Check sheet for the modelled part. Datum: model origin and axes. Units: mm. A direction names the side the tool comes from. Give positions to 0.01 mm unless a question says otherwise; leave off trailing zeros. Loops run counter-clockwise (first coordinate to the right, second up) from the corner with the lowest first, then second, coordinate; pieces in that order, holes last. Notation, with made-up numbers: (76, -24) - (87, -24) arc R19 cw to (87, 0) - close; hole circle Ø8 at (43.25, -23.75). An arc over 180 degrees is marked (long way). Use one line per item in the form item = value.
from build123d import *

# Parameters (mm, degrees)
SKETCH1_W           = 90
SKETCH1_H           = 80
BOSS_EXTRUDE1_DEPTH = 14
BOSS_EXTRUDE2_DEPTH = 1
SKETCH3_R           = 3.25
CUT_EXTRUDE1_DEPTH  = 111.613393245
SKETCH4_R           = 5.5
CUT_EXTRUDE2_DEPTH  = 7
SKETCH5_W           = 2
SKETCH5_H           = 6
SKETCH5_W_2         = 5
SKETCH5_H_2         = 5
CUT_EXTRUDE3_DEPTH  = 75
FILLET2_R           = 0.5
SKETCH6_R           = 1.5
CUT_EXTRUDE4_DEPTH  = 7
SKETCH7_R           = 1.5
CUT_EXTRUDE5_DEPTH  = 7
SKETCH8_W           = 12
SKETCH8_H           = 5
CUT_EXTRUDE6_DEPTH  = 5
SKETCH9_R           = 1.75
CUT_EXTRUDE7_DEPTH  = 111.09233745
SKETCH10_R          = 3
SKETCH10_R_2        = 3.25
CUT_EXTRUDE8_DEPTH  = 4
MOVE_FACE1_BY       = 0.2
MOVE_FACE1_2_BY     = 0.2
SKETCH11_W          = 10
SKETCH11_H          = 10
CUT_EXTRUDE10_DEPTH = 111.613393245


with BuildPart() as part:
    # Sketch1 → Boss-Extrude1 (new body)
    with BuildSketch(Plane(origin=(0, 0, 0), x_dir=(1, 0, 0), z_dir=(0, 1, 0))):
        with Locations((32.137715261, -38.032657583)):
            Rectangle(SKETCH1_W, SKETCH1_H)
    extrude(amount=BOSS_EXTRUDE1_DEPTH)

    # Sketch2 → Boss-Extrude2 (add)
    with BuildSketch(Plane(origin=(0, 14, 0), x_dir=(1, 0, 0), z_dir=(0, 1, 0))):
        Polygon((-12.862284739, -78.032657583), (77.137715261, -78.032657583), (77.137715261, -68.032657583), (77.137715261, 1.967342417), (70.137715261, 1.967342417), (70.137715261, -73.032657583), (-5.862284739, -73.032657583), (-5.862284739, 1.967342417), (-12.862284739, 1.967342417), (-12.862284739, -73.032657583), align=None)
    extrude(amount=BOSS_EXTRUDE2_DEPTH)

    # Sketch3 → Cut-Extrude1 (cut, through all)
    with BuildSketch(Plane(origin=(0, 14, 0), x_dir=(1, 0, 0), z_dir=(0, 1, 0))):
        with Locations(Location((57.137715261, -38.032657583, 0), (0, 0, 270))):
            Circle(SKETCH3_R)
        with Locations(Location((7.137715261, -38.032657583, 0), (0, 0, 270))):
            Circle(SKETCH3_R)
        with Locations(Location((7.137715261, -13.032657583, 0), (0, 0, 270))):
            Circle(SKETCH3_R)
        with Locations(Location((57.137715261, -13.032657583, 0), (0, 0, 270))):
            Circle(SKETCH3_R)
    extrude(amount=-CUT_EXTRUDE1_DEPTH, mode=Mode.SUBTRACT)

    # Sketch4 → Cut-Extrude2 (cut)
    with BuildSketch(Plane(origin=(0, 14, 0), x_dir=(1, 0, 0), z_dir=(0, 1, 0))):
        with Locations(Location((7.137715261, -38.032657583, 0), (0, 0, 270))):
            Circle(SKETCH4_R)
        with Locations(Location((57.137715261, -38.032657583, 0), (0, 0, 270))):
            Circle(SKETCH4_R)
        with Locations(Location((57.137715261, -13.032657583, 0), (0, 0, 270))):
            Circle(SKETCH4_R)
        with Locations(Location((7.137715261, -13.032657583, 0), (0, 0, 270))):
            Circle(SKETCH4_R)
    extrude(amount=-CUT_EXTRUDE2_DEPTH, mode=Mode.SUBTRACT)

    # Sketch5 → Cut-Extrude3 (cut)
    with BuildSketch(Plane(origin=(0, 0, -1.967342417), x_dir=(-1, 0, 0), z_dir=(0, 0, -1))):
        Polygon((-45.637715261, 14), (-43.637715261, 14), (-39.637715261, 10), (-49.637715261, 10), align=None)
        Polygon((-14.637715261, 10), (-24.637715261, 10), (-20.637715261, 14), (-18.637715261, 14), align=None)
        with Locations((-69.137715261, 11)):
            Rectangle(SKETCH5_W, SKETCH5_H)
        with Locations((4.862284739, 11)):
            Rectangle(SKETCH5_W, SKETCH5_H)
        with Locations((-32.137715261, 11.5)):
            Rectangle(SKETCH5_W_2, SKETCH5_H_2)
    extrude(amount=-CUT_EXTRUDE3_DEPTH, mode=Mode.SUBTRACT)

    # Fillet2
    fillet2_edges = [part.edges().sort_by_distance(p)[0] for p in [
        (68.137715261, 14, 35.532657583),
        (-3.862284739, 14, 35.532657583),
        (20.637715261, 14, 35.532657583),
        (18.637715261, 14, 35.532657583),
        (43.637715261, 14, 35.532657583),
        (45.637715261, 14, 35.532657583),
    ]]
    fillet(fillet2_edges, radius=FILLET2_R)

    # Sketch6 → Cut-Extrude4 (cut)
    with BuildSketch(Plane(origin=(77.137715261, 0, 0), x_dir=(0, 0, -1), z_dir=(1, 0, 0))):
        with Locations((-3.032657583, 12.5)):
            Circle(SKETCH6_R)
        with Locations((-13.032657583, 12.5)):
            Circle(SKETCH6_R)
        with Locations((-23.032657583, 12.5)):
            Circle(SKETCH6_R)
        with Locations((-33.032657583, 12.5)):
            Circle(SKETCH6_R)
        with Locations((-43.032657583, 12.5)):
            Circle(SKETCH6_R)
        with Locations((-53.032657583, 12.5)):
            Circle(SKETCH6_R)
        with Locations((-63.032657583, 12.5)):
            Circle(SKETCH6_R)
    extrude(amount=-CUT_EXTRUDE4_DEPTH, mode=Mode.SUBTRACT)

    # Sketch7 → Cut-Extrude5 (cut)
    with BuildSketch(Plane.ZY.offset(12.862284739)):
        with Locations((3.032657583, 11)):
            Circle(SKETCH7_R)
        with Locations((13.032657583, 11)):
            Circle(SKETCH7_R)
        with Locations((23.032657583, 11)):
            Circle(SKETCH7_R)
        with Locations((33.032657583, 11)):
            Circle(SKETCH7_R)
        with Locations((43.032657583, 11)):
            Circle(SKETCH7_R)
        with Locations((53.032657583, 11)):
            Circle(SKETCH7_R)
        with Locations((63.032657583, 11)):
            Circle(SKETCH7_R)
    extrude(amount=-CUT_EXTRUDE5_DEPTH, mode=Mode.SUBTRACT)

    # Sketch8 → Cut-Extrude6 (cut)
    with BuildSketch(Plane(origin=(0, 0, -1.967342417), x_dir=(-1, 0, 0), z_dir=(0, 0, -1))):
        with Locations((-32.137715261, 11.5)):
            Rectangle(SKETCH8_W, SKETCH8_H)
    extrude(amount=-CUT_EXTRUDE6_DEPTH, mode=Mode.SUBTRACT)

    # Sketch9 → Cut-Extrude7 (cut, through all)
    with BuildSketch(Plane(origin=(0, 9, 0), x_dir=(1, 0, 0), z_dir=(0, 1, 0))):
        with Locations(Location((36.137715261, -0.532657583, 0), (0, 0, 270))):
            Circle(SKETCH9_R)
        with Locations(Location((28.137715261, -0.532657583, 0), (0, 0, 90))):
            Circle(SKETCH9_R)
    extrude(amount=-CUT_EXTRUDE7_DEPTH, mode=Mode.SUBTRACT)

    # Sketch10 → Cut-Extrude8 (cut)
    with BuildSketch(Plane.XZ):
        with Locations((36.137715261, 0.532657583)):
            Circle(SKETCH10_R)
        with Locations((28.137715261, 0.532657583)):
            Circle(SKETCH10_R_2)
    extrude(amount=-CUT_EXTRUDE8_DEPTH, mode=Mode.SUBTRACT)

    # Move Face1: a face moved inward by 0.2
    extrude(part.faces().sort_by_distance((70.137715261, 11.395945296, 35.792794344))[0], amount=MOVE_FACE1_BY, dir=(1, 0, 0), mode=Mode.SUBTRACT)

    # Move Face1 2: a face moved inward by 0.2
    extrude(part.faces().sort_by_distance((-5.862284739, 11.552027352, 35.792794344))[0], amount=MOVE_FACE1_2_BY, dir=(-1, 0, 0), mode=Mode.SUBTRACT)

    # Sketch11 → Cut-Extrude10 (cut, through all)
    with BuildSketch(Plane(origin=(0, 14, 0), x_dir=(1, 0, 0), z_dir=(0, 1, 0))):
        with Locations((7.03416187, -63.032657583)):
            Rectangle(SKETCH11_W, SKETCH11_H)
        with Locations((57.241268652, -63.032657583)):
            Rectangle(SKETCH11_W, SKETCH11_H)
    extrude(amount=-CUT_EXTRUDE10_DEPTH, mode=Mode.SUBTRACT)


solid = part.part
Item 1: Gauge pin test, flat ends, axial feed: P1, Ø14.5, axis at x = 57.14, z = 13.03, coming from the +Y side; P2, Ø5.5, axis at x = 28.14, z = 0.53, coming from the -Y side; P3, Ø1.8, axis at y = 12.5, z = 63.03, coming from the +X side. Record the tip position at first contact, or that the pin passes through.
Answer block:
P1 = 14
P2 = 4
P3 = 68.14
Item 2: Access from +Z, -Z, +X, -X, +Y, -Y to the whole of each face (thin tool, end or side, straight path). Record for faces 1 (the face through (29.638, 11, 38)), 2 (the face through (74, 11, 3)), 3 (the face through (2.034, 7, 63)).
Answer block:
face_1 = -Z, +Y
face_2 = +X
face_3 = +Y, -Y
Item 3: Thickness scan on L1, parallel to X at y = 8.75, z = 28; L2, parallel to X at y = 1.25, z = 59; L3, parallel to X at y = 13.5, z = 21. Record the ranges inside material, lowest first.
Answer block:
L1 = -12.86 to -6.06, -3.86 to 68.14, 70.34 to 77.14
L2 = -12.86 to 2.03, 12.03 to 52.24, 62.24 to 77.14
L3 = -12.86 to -6.06, -3.86 to 17.93, 21.34 to 29.64, 34.64 to 42.93, 46.34 to 68.14, 70.34 to 77.14
Item 4: Mould release check, pull along X, two halves, no side actions. Record for faces 4 (the face through (32, 13, 73.033)), 5 (the face through (73.785, 11.925, 11.647)): released by +X, released by -X, zero draft, split by the parting line, or undercut.
Answer block:
face_4 = undercut
face_5 = zero draft
Item 5: Section check A-A on y = 2.25. Record the boundary of the cut face in (x, z), then the cut area to 3 significant figures.
Answer block:
outline = (-12.86, -1.97) - (26.06, -1.97) arc R3.25 cw (long way) to (30.21, -1.97) - (34.48, -1.97) arc R3 cw (long way) to (37.8, -1.97) - (77.14, -1.97) - (77.14, 78.03) - (-12.86, 78.03) - close; hole (2.03, 58.03) - (12.03, 58.03) - (12.03, 68.03) - (2.03, 68.03) - close; hole circle Ø6.5 at (7.14, 13.03); hole circle Ø6.5 at (7.14, 38.03); hole (52.24, 58.03) - (62.24, 58.03) - (62.24, 68.03) - (52.24, 68.03) - close; hole circle Ø6.5 at (57.14, 13.03); hole circle Ø6.5 at (57.14, 38.03)
area = 6,810 mm2
